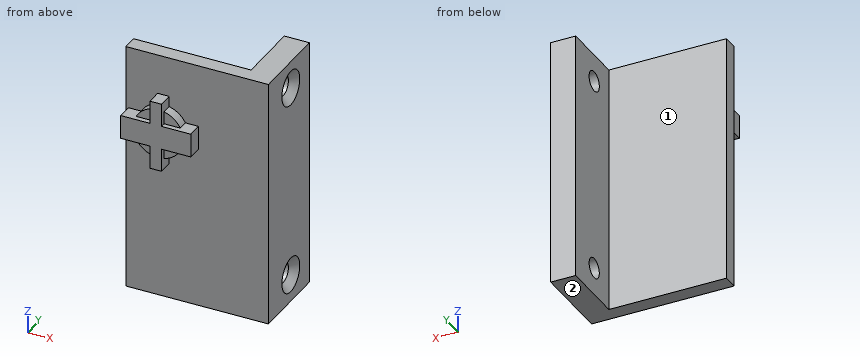
from build123d import *

# Parameters (mm, degrees)
SKETCH020_W       = 2.3
SKETCH020_H       = 14
PAD010_DEPTH      = 3
SKETCH021_W       = 14
SKETCH021_H       = 4.75
PAD011_DEPTH      = 3
SKETCH022_R       = 5
PAD012_DEPTH      = 2
SKETCH023_W       = 28.5
SKETCH023_H       = 50
PAD013_DEPTH      = 3
SKETCH024_W       = 5
SKETCH024_H       = 50
PAD014_DEPTH      = 13
CYLINDER003_R     = 2
CYLINDER003_DEPTH = 15
CHAMFER001_SIZE   = 1.5


with BuildPart() as part:
    # Sketch020 → Pad010 (new body)
    with BuildSketch(Plane.XZ.offset(3)):
        with Locations((0, 10)):
            Rectangle(SKETCH020_W, SKETCH020_H)
    extrude(amount=PAD010_DEPTH)

    # Sketch021 → Pad011 (join)
    with BuildSketch(Plane.XZ.offset(3)):
        with Locations((0, 9.995)):
            Rectangle(SKETCH021_W, SKETCH021_H)
    extrude(amount=PAD011_DEPTH)

    # Sketch022 → Pad012 (join)
    with BuildSketch(Plane.XZ.offset(3)):
        with Locations((0, 10)):
            Circle(SKETCH022_R)
    extrude(amount=PAD012_DEPTH)

    # Sketch023 → Pad013 (join)
    with BuildSketch(Plane.XZ):
        with Locations((6.75, 0)):
            Rectangle(SKETCH023_W, SKETCH023_H)
    extrude(amount=PAD013_DEPTH)

    # Sketch024 → Pad014 (join)
    with BuildSketch(Plane.XZ):
        with Locations((18.5, 0)):
            Rectangle(SKETCH024_W, SKETCH024_H)
    extrude(amount=-PAD014_DEPTH)

    # Cylinder003 → Cylinder003 (cut)
    with BuildSketch(Plane(origin=(10, 5.75, -19.5), x_dir=(0, 1, 0), z_dir=(1, 0, 0))):
        Circle(CYLINDER003_R)
    cylinder003 = extrude(amount=CYLINDER003_DEPTH, mode=Mode.SUBTRACT)

    # Mirrored011: Cylinder003 across XY
    add(cylinder003.mirror(Plane.XY), mode=Mode.SUBTRACT)

    # Chamfer001
    chamfer001_edges = [part.edges().sort_by_distance(p)[0] for p in [
        (21, 3.75, -19.5),
        (21, 3.75, 19.5),
    ]]
    chamfer(chamfer001_edges, length=CHAMFER001_SIZE)


solid = part.part
The listing builds one solid part. Answer for the finished solid, in the listing's coordinates (mm). Face numbers are marked on the shaded views. A direction names the side the tool comes from. Round coordinates to 2 decimals unless told otherwise and drop trailing zeros. Order: outer loops, then holes, each group sorted by start corner. A loop starts at its lowest first (then second) coordinate and runs counter-clockwise, first axis right, second up. Notation, with made-up numbers: (6, -32.75) - (23, -32.75) arc R29 ccw to (23, -7.75) - close; hole circle Ø7 at (41, -25). An arc over 180 degrees is marked (long way). Write item = value, one per line. Start each with the question number.
1) Straight lines are drawn through the part: L1, parallel to Z at x = 17.4, y = 5.75; L2, parallel to Y at x = 18.65, z = 19.5; L3, parallel to Y at x = 10.75, z = -6.5. For each, find the intervals that lie inside material, in ascending order.
2) Section B-B, the plane z = -19.5 is taken. Write down the section's boundary in (x, y).
3) Given pin 1 (2.5 mm diameter, centred on x = 3.5, z = 7, fed in from -Y); pin 2 (1.5 mm diameter, centred on x = 5.5, y = -4, fed in from -Z); pin 3 (5 mm diameter, centred on y = 9, z = -9.5, fed in from -X); pin 4 (2.5 mm diameter, centred on x = -5, y = -4.5, fed in from -Z), each flat-ended and moving along its own axis, determine where each tip first touches the part or whether it passes through.
4) Section A-A, the plane y = 5.75 is taken. Write down the section's boundary in (x, z), plus the area to 4 significant figures.
5) Section D-D, the plane z = 9 is taken. Write down the section's boundary in (x, y).
6) Section C-C, the plane x = 5 is taken. Write down the section's boundary in (y, z).
7) For the marked faces 1 and 2, determine the directions among +Z, -Z, +X, -X, +Y, -Y from which every point of the face is accessible in a straight line to the end or side of a thin tool.
Results list:
q1.L1 = -25 to -21.5, -17.5 to 17.5, 21.5 to 25
q1.L2 = -3 to 3.75, 7.75 to 13
q1.L3 = -3 to 0
q2.outline = (-7.5, -3) - (21, -3) - (21, 2.25) - (19.5, 3.75) - (16, 3.75) - (16, 0) - (-7.5, 0) - close; (16, 7.75) - (19.5, 7.75) - (21, 9.25) - (21, 13) - (16, 13) - close
q3.pin_1 = -6
q3.pin_2 = 7.62
q3.pin_3 = 16
q3.pin_4 = 6.69
q4.outline = (16, -25) - (21, -25) - (21, -23) - (19.5, -21.5) - (16, -21.5) - close; (16, -17.5) - (19.5, -17.5) - (21, -16) - (21, 16) - (19.5, 17.5) - (16, 17.5) - close; (16, 21.5) - (19.5, 21.5) - (21, 23) - (21, 25) - (16, 25) - close
q4.area = 205.5 mm^2
q5.outline = (-7.5, -3) - (-7, -3) - (-7, -6) - (7, -6) - (7, -3) - (21, -3) - (21, 13) - (16, 13) - (16, 0) - (-7.5, 0) - close
q6.outline = (-6, 7.62) - (-3, 7.62) - (-3, -25) - (0, -25) - (0, 25) - (-3, 25) - (-3, 12.37) - (-6, 12.37) - close
q7.face_1 = +Z, -Z, -X, +Y
q7.face_2 = -Z, +X, -X, +Y, -Y
